Geometry check sheet. Reference: the model listing, model coordinates, mm. A direction names the side the tool comes from. Coordinates: 2 decimals unless noted, no trailing zeros. Write each loop counter-clockwise with the first axis right and the second up, starting at its lowest first coordinate (ties: lowest second). Pieces come first, ordered by that corner, then holes. Notation, with made-up numbers: (-37.5, -10.5) -> (8.5, -10.5) arc R10 cw to (8.5, -2.5) -> close; hole circle Ø1 at (9, 71.25). An arc over 180 degrees is marked (long way). Use a Markdown table: item, result.
Autodesk Inventor part; units mm, degrees
ref_plane "YZ Plane" through (0, 0, 0) normal (1, 0, 0) x (0, 1, 0)
ref_plane "XZ Plane" through (0, 0, 0) normal (0, 1, 0) x (-1, 0, 0)
ref_plane "XY Plane" through (0, 0, 0) normal (0, 0, 1) x (1, 0, 0)
sketch "Sketch1" plane through (0, 0, 0) normal (0, 0, 1) x (1, 0, 0)
  line L0 (-12.7, -12.7) -> (12.7, -12.7)
  line L1 (12.7, -12.7) -> (12.7, 12.7)
  line L2 (12.7, 12.7) -> (-12.7, 12.7)
  line L3 (-12.7, 12.7) -> (-12.7, -12.7)
  line L4 (-12.7, -12.7) -> (12.7, 12.7) construction
  line L5 (12.7, -12.7) -> (-12.7, 12.7) construction
  line L6 (-9.525, -9.525) -> (9.525, -9.525)
  line L7 (9.525, -9.525) -> (9.525, 9.525)
  line L8 (9.525, 9.525) -> (-9.525, 9.525)
  line L9 (-9.525, 9.525) -> (-9.525, -9.525)
  line L10 (-9.525, -9.525) -> (9.525, 9.525) construction
  line L11 (9.525, -9.525) -> (-9.525, 9.525) construction
  point P0 (0, 0)
  dimension "d0" = 25.4
  dimension "d1" = 25.4
  dimension "d2" = 3.175
extrude "Extrusion1" add sketch "Sketch1" along normal mid plane 239.7125
sketch "Sketch4" plane through (12.7, -12.7, 119.8563) normal (1, 0, 0) x (0, 0, -1)
  line L0 (239.7125, 0) -> (239.7125, 25.4)
  line L1 (239.7125, 0) -> (218.3994, 25.4)
  line L2 (239.7125, 25.4) -> (0, 25.4)
  line L3 (218.3994, 25.4) -> (239.7125, 25.4)
  line L4 (0, 22.225) -> (239.7125, 22.225)
  line L5 (239.7125, 25.4) -> (239.7125, 0)
  point P0 (119.8563, 12.7)
  dimension "d9" = 40
extrude "Extrusion3" cut sketch "Sketch4" against normal through all
properties part number "Aluminum1x1MiddleFront" material "Aluminum 6061"
Item 1: Mould release check, pull along X, two halves, no side actions. Record for faces 1 (the flat face through (-9.525, 0, 0)), 2 (the flat face through (0, 12.7, 9)), 3 (the flat face through (-12.7, 0, -2)): +X half, -X half, draft (parallel to the pull), parting line (faces both ways), or undercut.
Answer block:
| item | result |
|---|---|
| face 1 | undercut |
| face 2 | draft |
| face 3 | -X half |
Item 2: Tool access check on faces 4 (the flat face through (12.7, 0, -2)), 5 (the flat face through (0, -9.525, 0)). Record the directions out of +Z, -Z, +X, -X, +Y, -Y that give a thin tool (end or side, any length) a straight path to the whole face; none if there is none.
Answer block:
| item | result |
|---|---|
| face 4 | +Z, -Z, +X, +Y, -Y |
| face 5 | +Z, -Z |
Item 3: Section check B-B on z = 6. Record the boundary of the cut face in (x, y) (3 decimals).
Answer block:
| item | result |
|---|---|
| outline | (-12.7, -12.7) -> (12.7, -12.7) -> (12.7, 12.7) -> (-12.7, 12.7) -> close; hole (-9.525, -9.525) -> (9.525, -9.525) -> (9.525, 9.525) -> (-9.525, 9.525) -> close |
Item 4: Section check A-A on x = 6.5. Record the boundary of the cut face in (y, z) (3 decimals).
Answer block:
| item | result |
|---|---|
| outline | (-12.7, -119.856) -> (-9.525, -117.192) -> (-9.525, 119.856) -> (-12.7, 119.856) -> close; (9.525, -101.207) -> (12.7, -98.543) -> (12.7, 119.856) -> (9.525, 119.856) -> close |
Item 5: Thickness scan on L1, parallel to Y at x = -6, z = -7 (3 decimals); L2, parallel to Z at x = -11.5, y = -11.5. Record the ranges inside material, lowest first. Write a range as [from, to].
Answer block:
| item | result |
|---|---|
| L1 | y = [-12.7, -9.525], [9.525, 12.7] |
| L2 | z = [-118.85, 119.86] |
Item 6: Section check C-C on y = -2. Record the boundary of the cut face in (x, z) (3 decimals).
Answer block:
| item | result |
|---|---|
| outline | (-12.7, -110.878) -> (-9.525, -110.878) -> (-9.525, 119.856) -> (-12.7, 119.856) -> close; (9.525, -110.878) -> (12.7, -110.878) -> (12.7, 119.856) -> (9.525, 119.856) -> close |
